Study the drawing (mm; zero at the part's minimum x, y, z) and answer. Give positions to 0.01 mm unless a question says otherwise; leave off trailing zeros. Loops run counter-clockwise (first coordinate to the right, second up) from the corner with the lowest first, then second, coordinate; pieces in that order, holes last. Notation, with made-up numbers: M 44,74.25 L 62,74.25 A14 ccw 62,82.25 Z; hole C 77,70.5 d2. An arc over 180 degrees is marked long. Return JSON: item names as keys, results as strings.
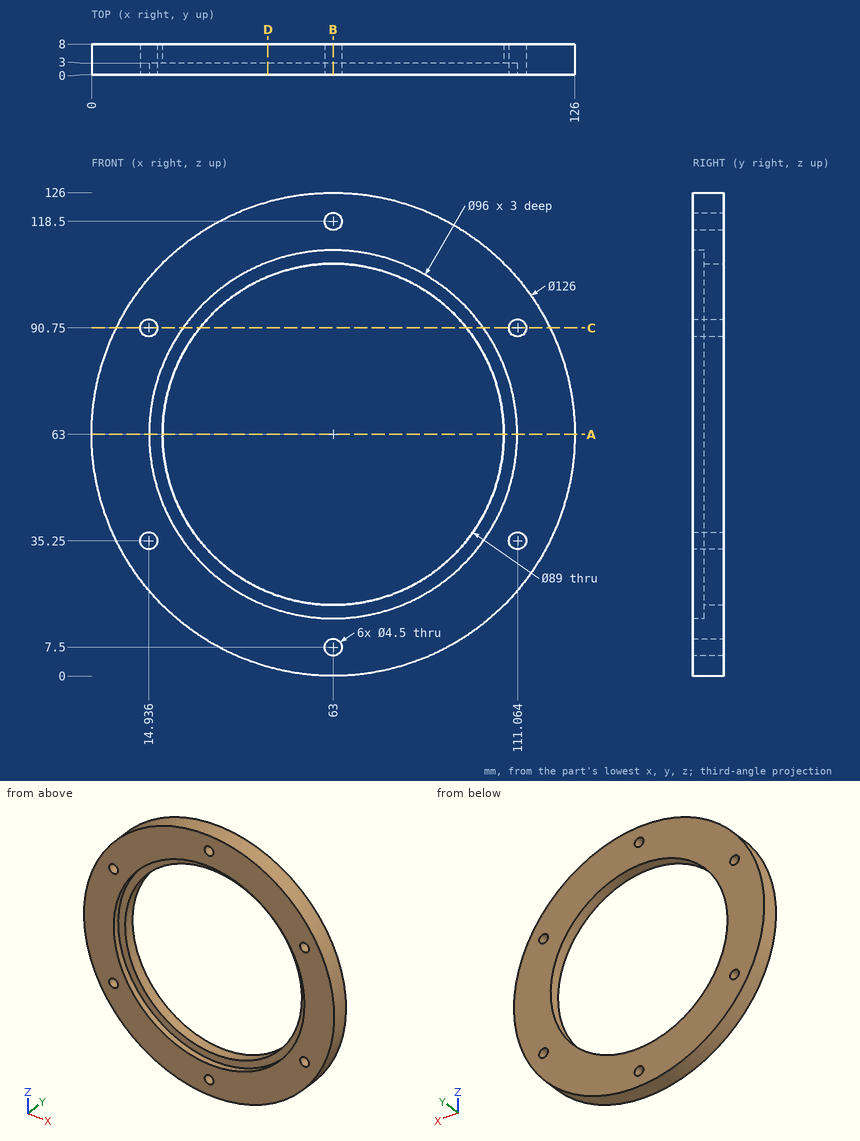
(1) The part is cut by section C-C (z = 90.75). Determine the outline of the cut face in (x, y) (1 decimal), and give its area (3 significant figures).
Values follow:
{"outline": "M 6.4,0 L 12.7,0 L 12.7,8 L 6.4,8 Z; M 17.2,0 L 23.8,0 L 23.8,3 L 28.2,3 L 28.2,8 L 17.2,8 Z; M 97.8,3 L 102.2,3 L 102.2,0 L 108.8,0 L 108.8,8 L 97.8,8 Z; M 113.3,0 L 119.6,0 L 119.6,8 L 113.3,8 Z", "area": "250 mm²"}
(2) Given pin 1 (2 mm diameter, centred on x = 71, y = 2, fed in from +Z); pin 2 (3 mm diameter, centred on x = 23.5, y = 5.5, fed in from -Z); pin 3 (3 mm diameter, centred on y = 1, z = 32, fed in from +X); pin 4 (3.5 mm diameter, centred on x = 111.06, z = 35.25, fed in from +Y), each flat-ended and moving along its own axis, determine where each tip first touches the part or whether it passes through.
Values follow:
{"pin 1": "z = 125.61", "pin 2": "z = 12.75", "pin 3": "x = 118.67", "pin 4": "through"}
(3) The part is cut by section D-D (x = 46). Determine the outline of the cut face in (y, z) (1 decimal).
Values follow:
{"outline": "M 0,2.3 L 8,2.3 L 8,21.9 L 3,21.9 L 3,18.1 L 0,18.1 Z; M 0,107.9 L 3,107.9 L 3,104.1 L 8,104.1 L 8,123.7 L 0,123.7 Z"}
(4) Straight lines are drawn through the part: line 1 along X through (y, z) = (2, 63.5); line 2 along X through (y, z) = (5.15, 63); line 3 along X through (y, z) = (3.5, 90.75) (1 decimal). For each, find the intervals that lie inside material, in ascending order.
Values follow:
{"line 1": "0 to 15, 111 to 126", "line 2": "0 to 18.5, 107.5 to 126", "line 3": "6.4 to 12.7, 17.2 to 28.2, 97.8 to 108.8, 113.3 to 119.6"}
(5) The part is cut by section B-B (x = 63). Determine the outline of the cut face in (y, z), and give its area (3 significant figures).
Values follow:
{"outline": "M 0,0 L 8,0 L 8,5.25 L 0,5.25 Z; M 0,9.75 L 8,9.75 L 8,18.5 L 3,18.5 L 3,15 L 0,15 Z; M 0,111 L 3,111 L 3,107.5 L 8,107.5 L 8,116.25 L 0,116.25 Z; M 0,120.75 L 8,120.75 L 8,126 L 0,126 Z", "area": "203 mm²"}
(6) The part is cut by section A-A (z = 63). Determine the outline of the cut face in (x, y), and give its area (3 significant figures).
Values follow:
{"outline": "M 0,0 L 15,0 L 15,3 L 18.5,3 L 18.5,8 L 0,8 Z; M 107.5,3 L 111,3 L 111,0 L 126,0 L 126,8 L 107.5,8 Z", "area": "275 mm²"}
